Geometry: final body of the model. Coordinates: model frame, mm. Face numbers are marked on the shaded views. Give positions to 0.01 mm unless a question says otherwise; leave off trailing zeros. Write each loop counter-clockwise with the first axis right and the second up, starting at its lowest first coordinate (ties: lowest second). Pieces come first, ordered by that corner, then holes.
Q1. Draft query along X for the marked faces 1, 2, 3 and 4. Return one class per face: pulls with the +X half, pulls with the -X half, needs draft (parallel to the pull), parting line crosses it, or undercut.
Q2. Line query: L1, parallel to X at y = 5.6, z = 3.5; L2, parallel to Y at x = -26, z = 3.25; L3, parallel to X at y = 14, z = 52.5. Output: solid intervals per line, ascending.
Q3. Pin query (flat end, axial travel): pin 1 (9 mm diameter, centred on x = -30.5, z = 17.5, fed in from +Y); pin 2 (1.9 mm diameter, centred on x = -26, y = 5.6, fed in from -Z); pin 3 (2.5 mm diameter, centred on x = -30, y = 15.5, fed in from -Z). Return the tip coordinate at first contact, or that it passes through.
Q4. Cut plane C-C on z = 54. Return the cut outline in (x, y).
Q5. Cut plane A-A on x = -31. Return the cut outline in (y, z), plus the area to 3 significant figures.
Q6. Cut plane B-B on y = 14.5. Return the cut outline in (x, z).
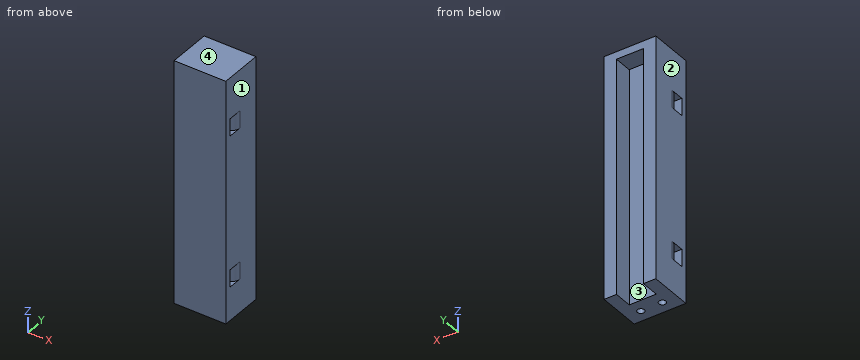
```python
from build123d import *

# Parameters (mm, degrees)
SKETCH1_W                 = 12.5
SKETCH1_H                 = 11.5
BOSS_EXTRUDE1_DEPTH       = 109
SKETCH2_W                 = 24
SKETCH2_H                 = 20
BOSS_EXTRUDE2_DEPTH       = 3.5
F_2_5MM_DOWEL_HOLE1_D     = 3.2
F_2_5MM_DOWEL_HOLE1_DEPTH = 6.5
F_2_5MM_DOWEL_HOLE1_TIP   = 0.96137699
SKETCH5_W                 = 8
SKETCH5_H                 = 2.5
CUT_EXTRUDE1_DEPTH        = 117.757226757
FILLET1_R                 = 4


with BuildPart() as part:
    # Sketch1 → Boss-Extrude1 (new body)
    with BuildSketch(Plane.XY):
        Polygon((-37.25, 0), (-37.25, 11.5), (-37.25, 20), (-43, 20), (-43, 0), align=None)
        with Locations((-31, 5.75)):
            Rectangle(SKETCH1_W, SKETCH1_H)
        Polygon((-24.75, 20), (-24.75, 11.5), (-24.75, 0), (-19, 0), (-19, 20), align=None)
    extrude(amount=BOSS_EXTRUDE1_DEPTH)

    # Sketch2 → Boss-Extrude2 (add)
    with BuildSketch(Plane.XY.offset(109)):
        with Locations((-31, 10)):
            Rectangle(SKETCH2_W, SKETCH2_H)
    extrude(amount=BOSS_EXTRUDE2_DEPTH)

    # Ø2.5mm Dowel Hole1
    with Locations(Plane(origin=(0, 0, 0), x_dir=(-1, 0, 0), z_dir=(0, 0, -1))):
        with Locations((36, 5.6), (26, 5.6)):
            Hole(F_2_5MM_DOWEL_HOLE1_D / 2, depth=F_2_5MM_DOWEL_HOLE1_DEPTH)
            with Locations((0, 0, -(F_2_5MM_DOWEL_HOLE1_DEPTH + F_2_5MM_DOWEL_HOLE1_TIP / 2))):  # 118° drill point
                Cone(0, F_2_5MM_DOWEL_HOLE1_D / 2, F_2_5MM_DOWEL_HOLE1_TIP, mode=Mode.SUBTRACT)

    # Sketch5 → Cut-Extrude1 (cut, through all)
    with BuildSketch(Plane(origin=(-19, 0, 0), x_dir=(0, 0, -1), z_dir=(1, 0, 0))):
        with Locations((-89.5, 4)):
            Rectangle(SKETCH5_W, SKETCH5_H)
        with Locations((-19.5, 4)):
            Rectangle(SKETCH5_W, SKETCH5_H)
    extrude(amount=-CUT_EXTRUDE1_DEPTH, mode=Mode.SUBTRACT)

    # Fillet1
    fillet1_edges = [part.edges().sort_by_distance(p)[0] for p in [
        (-43, 5.25, 89.5),
        (-19, 5.25, 89.5),
        (-43, 5.25, 19.5),
        (-19, 5.25, 19.5),
    ]]
    fillet(fillet1_edges, radius=FILLET1_R)


solid = part.part
```
Data:
1. face 1: pulls with the +X half
1. face 2: pulls with the -X half
1. face 3: undercut
1. face 4: needs draft
2. L1: x = -43 to -37.6, -34.4 to -27.6, -24.4 to -19
2. L2: y = 0 to 4, 7.2 to 11.5
2. L3: x = -43 to -37.25, -24.75 to -19
3. pin 1: stops at y = 11.5
3. pin 2: stops at z = 6.89
3. pin 3: stops at z = 109
4. outline: (-43, 0) - (-19, 0) - (-19, 20) - (-24.75, 20) - (-24.75, 11.5) - (-37.25, 11.5) - (-37.25, 20) - (-43, 20) - close
5. outline: (0, 0) - (11.5, 0) - (11.5, 109) - (20, 109) - (20, 112.5) - (0, 112.5) - close; hole (2.75, 15.5) - (5.25, 15.5) - (5.25, 23.5) - (2.75, 23.5) - close; hole (2.75, 85.5) - (5.25, 85.5) - (5.25, 93.5) - (2.75, 93.5) - close
5. area: 1,280 mm2
6. outline: (-43, 0) - (-37.25, 0) - (-37.25, 109) - (-24.75, 109) - (-24.75, 0) - (-19, 0) - (-19, 112.5) - (-43, 112.5) - close
